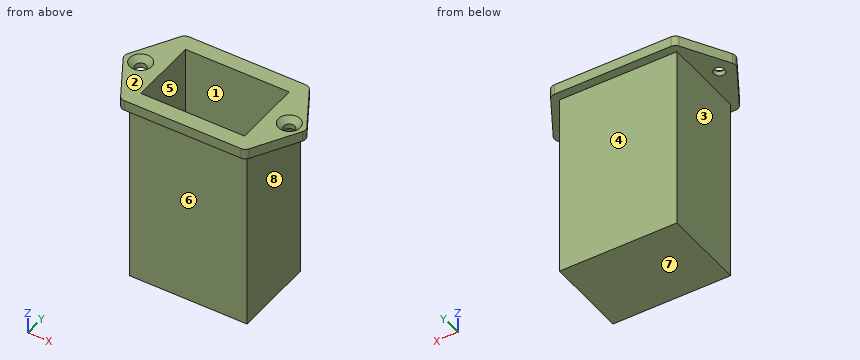
Autodesk Inventor part; units mm, degrees
ref_plane "YZ Plane" through (0, 0, 0) normal (1, 0, 0) x (0, 1, 0)
ref_plane "XZ Plane" through (0, 0, 0) normal (0, 1, 0) x (-1, 0, 0)
ref_plane "XY Plane" through (0, 0, 0) normal (0, 0, 1) x (1, 0, 0)
sketch "Sketch1" plane through (0, 0, 0) normal (0, 0, 1) x (1, 0, 0)
  line L0 (-25.9071, 1.0114) -> (-18.5795, 13.5114)
  line L1 (-16.8541, 14.5) -> (16.8541, 14.5)
  line L2 (18.5795, 13.5114) -> (25.9071, 1.0114)
  arc A0 (-16.8541, 14.5) -> (-18.5795, 13.5114) centre (-16.8541, 12.5) ccw
  arc A1 (18.5795, 13.5114) -> (16.8541, 14.5) centre (16.8541, 12.5) ccw
  line L3 (-28.1394, 0) -> (29.237, 0) construction
  line L4 (-25.9071, -1.0114) -> (-18.5795, -13.5114)
  line L5 (-16.8541, -14.5) -> (16.8541, -14.5)
  line L6 (18.5795, -13.5114) -> (25.9071, -1.0114)
  arc A2 (-18.5795, -13.5114) -> (-16.8541, -14.5) centre (-16.8541, -12.5) ccw
  arc A3 (16.8541, -14.5) -> (18.5795, -13.5114) centre (16.8541, -12.5) ccw
  arc A4 (-25.9071, 1.0114) -> (-25.9071, -1.0114) centre (-24.1817, 0) ccw
  arc A5 (25.9071, -1.0114) -> (25.9071, 1.0114) centre (24.1817, 0) ccw
  point P0 (0, 0)
  point P1 (-26.5, 0)
  point P2 (-18, 14.5)
  point P3 (18, 14.5)
  point P4 (26.5, 0)
  point P5 (-18, -14.5)
  point P6 (18, -14.5)
  dimension "d0" = 53
  dimension "d1" = 26.5
  dimension "d2" = 14.5
  dimension "d3" = 36
  dimension "d4" = 18
  dimension "d5" = 2
  dimension "d6" = 2
extrude "Extrusion1" add sketch "Sketch1" against normal blind 3
sketch "Sketch2" plane through (0, 0, 0) normal (0, 0, 1) x (1, 0, 0)
  point P0 (0, 0)
  point P1 (-21.5, 0)
  point P2 (21.5, 0)
  dimension "d9" = 43
  dimension "d10" = 21.5
hole "Hole1" at (-21.5, 0, 0) at (21.5, 0, 0) direction (0, 0, -1) diameter 3.2 end through all countersink diameter 6.35 countersink angle 90
sketch "Sketch3" plane through (0, 0, -3) normal (0, 0, -1) x (-1, 0, 0)
  line L0 (-17, 12) -> (17, 12)
  line L1 (17, 12) -> (17, -12)
  line L2 (17, -12) -> (-17, -12)
  line L3 (-17, -12) -> (-17, 12)
  point P0 (0, 0)
  dimension "d18" = 24
  dimension "d19" = 34
  dimension "d20" = 17
  dimension "d21" = 12
extrude "Extrusion2" add sketch "Sketch3" along normal blind 54
sketch "Sketch4" plane through (0, 0, 0) normal (0, 0, 1) x (1, 0, 0)
  line L0 (-15, 10) -> (15, 10)
  line L1 (15, 10) -> (15, -10)
  line L2 (15, -10) -> (-15, -10)
  line L3 (-15, -10) -> (-15, 10)
  point P0 (0, 0)
  dimension "d24" = 30
  dimension "d25" = 20
  dimension "d26" = 15
  dimension "d27" = 10
extrude "Extrusion3" cut sketch "Sketch4" against normal blind 49
properties part number "BatteryHolder_DigiKEY" material "ABS Plastic"
Can you work these out from the model? Positions are in its coordinate system, mm. Face numbers are marked on the shaded views. A direction names the side the tool comes from. Give positions to 0.01 mm unless a question says otherwise; leave off trailing zeros. Loops run counter-clockwise (first coordinate to the right, second up) from the corner with the lowest first, then second, coordinate; pieces in that order, holes last. Notation, with made-up numbers: (12, -2.5) - (27, -2.5) arc R19 ccw to (27, 2.5) - close; hole circle Ø9 at (84.25, 71.5). An arc over 180 degrees is marked (long way). Return JSON: item names as keys, results as strings.
1. For the marked faces 4, 5, 6, 7 and 8, which set-ups out of +Z, -Z, +X, -X, +Y, -Y let a thin tool reach every point of the face, with its end or its side?
Output values:
{"face 4": "-Z, +X, -X, +Y", "face 5": "+Z", "face 6": "-Z, +X, -X, -Y", "face 7": "-Z, +X, -X, +Y, -Y", "face 8": "-Z, +X, +Y, -Y"}
2. We'd pull the mould along X, two halves only. Please class the marked faces 1, 2 and 3: +X half, -X half, draft (parallel to the pull), parting line (faces both ways), or undercut.
Output values:
{"face 1": "undercut", "face 2": "draft", "face 3": "-X half"}
3. I want a section at C-C on x = -1. Please give me the cut outline in (y, z), and give its area (3 significant figures).
Output values:
{"outline": "(-14.5, -3) - (-12, -3) - (-12, -57) - (12, -57) - (12, -3) - (14.5, -3) - (14.5, 0) - (10, 0) - (10, -49) - (-10, -49) - (-10, 0) - (-14.5, 0) - close", "area": "403 mm²"}
4. I want a section at D-D on x = -21.5. Please give me the cut outline in (y, z) (3 decimals), and give its area (3 significant figures).
Output values:
{"outline": "(-8.529, -3) - (-1.6, -3) - (-1.6, -1.575) - (-3.175, 0) - (-8.529, 0) - close; (1.6, -3) - (8.529, -3) - (8.529, 0) - (3.175, 0) - (1.6, -1.575) - close", "area": "39.1 mm²"}
5. I want a section at B-B on y = 0. Please give me the cut outline in (x, z) (3 decimals).
Output values:
{"outline": "(-26.182, -3) - (-23.1, -3) - (-23.1, -1.575) - (-24.675, 0) - (-26.182, 0) - close; (-19.9, -3) - (-17, -3) - (-17, -57) - (17, -57) - (17, -3) - (19.9, -3) - (19.9, -1.575) - (18.325, 0) - (15, 0) - (15, -49) - (-15, -49) - (-15, 0) - (-18.325, 0) - (-19.9, -1.575) - close; (23.1, -3) - (26.182, -3) - (26.182, 0) - (24.675, 0) - (23.1, -1.575) - close"}
6. I'm going to push flat-ended pins straight in: pin 1 Ø5 at (y, z) = (-2.5, -15.5) entering from -X; pin 2 Ø12 at (x, z) = (-11, -43) entering from -Y; pin 3 Ø8 at (x, z) = (-7, -22.5) entering from +Y; pin 4 Ø1 at (x, y) = (-19.5, -9.5) entering from +Z. Where does each tip first touch, or does it pass through?
Output values:
{"pin 1": "stops at x = -17", "pin 2": "stops at y = -12", "pin 3": "stops at y = 12", "pin 4": "stops at z = 0"}
7. If I drill on line 1 (X direction, y = 9.25, z = -16); line 2 (Z direction, x = 12, y = -2.75); line 3 (Y direction, x = 1, z = -53.5), over which ranges is the centre line in solid material (lowest first)?
Output values:
{"line 1": "x = -17 to -15, 15 to 17", "line 2": "z = -57 to -49", "line 3": "y = -12 to 12"}
8. I want a section at A-A on z = -12.5. Please give me the cut outline in (x, y), and give its area (3 significant figures).
Output values:
{"outline": "(-17, -12) - (17, -12) - (17, 12) - (-17, 12) - close; hole (-15, -10) - (15, -10) - (15, 10) - (-15, 10) - close", "area": "216 mm²"}
